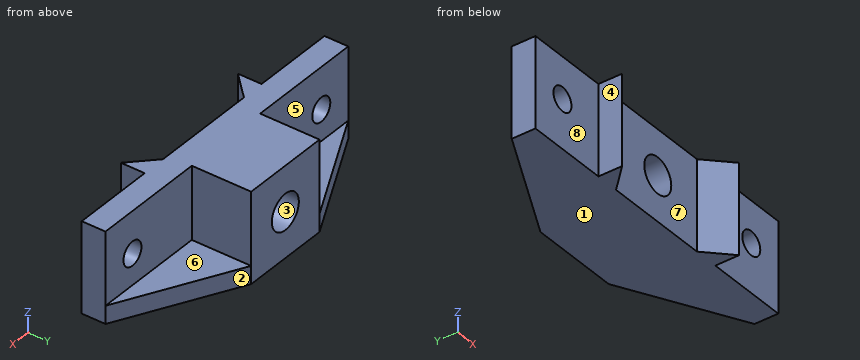
from build123d import *

# Parameters (mm, degrees)
BOSS_EXTRUDE1_DEPTH = 76
CUT_EXTRUDE1_DEPTH  = 61
SKETCH7_R           = 15
SKETCH7_R_2         = 10
CUT_EXTRUDE4_DEPTH  = 71


with BuildPart() as part:
    # Sketch2 → Boss-Extrude1 (new body)
    with BuildSketch(Plane.XY):
        Polygon((155.98455698, -34.815353078), (57.98455698, -84.815353078), (57.98455698, -104.815353078), (127.98455698, -104.815353078), (127.98455698, -124.815353078), (147.58455698, -104.815353078), (237.576393715, -104.815353078), (257.98455698, -124.815353078), (257.98455698, -104.815353078), (327.98455698, -104.815353078), (327.98455698, -84.815353078), (231.98455698, -34.815353078), align=None)
    extrude(amount=BOSS_EXTRUDE1_DEPTH)

    # Sketch5 → Cut-Extrude1 (cut)
    with BuildSketch(Plane.XY.offset(76)):
        Polygon((155.98455698, -34.815353078), (155.98455698, -84.815353078), (57.98455698, -84.815353078), align=None)
        Polygon((231.98455698, -34.815353078), (231.98455698, -84.815353078), (327.98455698, -84.815353078), align=None)
    extrude(amount=-CUT_EXTRUDE1_DEPTH, mode=Mode.SUBTRACT)

    # Sketch7 → Cut-Extrude4 (cut, through all)
    with BuildSketch(Plane(origin=(0, -104.815353078, 0), x_dir=(1, 0, 0), z_dir=(0, 1, 0))):
        with Locations((193.98455698, -38)):
            Circle(SKETCH7_R)
        with Locations((87.98455698, -41)):
            Circle(SKETCH7_R_2)
        with Locations((297.98455698, -41)):
            Circle(SKETCH7_R_2)
    extrude(amount=CUT_EXTRUDE4_DEPTH, mode=Mode.SUBTRACT)


solid = part.part
Model file for the job. Use its own axes, mm. Face numbers are marked on the shaded views. A direction names the side the tool comes from. Give positions to 0.01 mm unless a question says otherwise; leave off trailing zeros. Order: outer loops, then holes, each group sorted by start corner. A loop starts at its lowest first (then second) coordinate and runs counter-clockwise, first axis right, second up. Notation, with made-up numbers: M 20,24 L 25,24 A27 cw 25,54 Z; hole C 36,64 d9. An arc over 180 degrees is marked long. Put each result on its own line as item: value. Start each with the question number.
(1) Tool access for the marked faces 5, 6, 7 and 8: list every direction of +Z, -Z, +X, -X, +Y, -Y with a clear straight run to the whole face (end or side of a thin tool).
(2) Band-saw the part on A-A on z = 9. Give the cut face in (x, y), then the cut area to 3 significant figures.
(3) Band-saw the part on B-B on x = 190. Give the cut face in (y, z), then the cut area to 3 significant figures.
(4) Drill centre lines: L1, parallel to X at y = -90.75, z = 41; L2, parallel to X at y = -98, z = 49.5; L3, parallel to X at y = -115.5, z = 37. Where is each one in solid material? Low to high. Write a range as [from, to].
(5) Pin check, flat tips, straight feed: pin 1 Ø22 at (y, z) = (-119, 29) entering from -X; pin 2 Ø5 at (x, z) = (262, 12.5) entering from -Y; pin 3 Ø8 at (x, z) = (252.5, 53.5) entering from +Y. Stop position of each tip, or through.
(6) Band-saw the part on C-C on y = -58.5. Give the cut face in (x, z), then the cut area to 3 significant figures.
(7) Band-saw the part on D-D on z = 48.5. Give the cut face in (x, y), then the cut area to 3 significant figures.
(8) Pull direction X, two halves, no side cores. Call the marked faces 1, 2, 3 and 4: released by +X, released by -X, zero draft, split by the parting line, or undercut.
Results below:
1. face 5: +Z, -X, +Y
1. face 6: +Z, +X, +Y
1. face 7: +Z, -Z, -Y
1. face 8: +Z, -Z, -X, -Y
2. outline: M 57.98,-104.82 L 127.98,-104.82 L 127.98,-124.82 L 147.58,-104.82 L 237.58,-104.82 L 257.98,-124.82 L 257.98,-104.82 L 327.98,-104.82 L 327.98,-84.82 L 231.98,-34.82 L 155.98,-34.82 L 57.98,-84.82 Z
2. area: 14,500 mm2
3. outline: M -104.82,0 L -34.82,0 L -34.82,23.54 L -104.82,23.54 Z; M -104.82,52.46 L -34.82,52.46 L -34.82,76 L -104.82,76 Z
3. area: 3,300 mm2
4. L1: x = [57.98, 77.98], [97.98, 179.29], [208.68, 287.98], [307.98, 327.98]
4. L2: x = [57.98, 82.72], [93.25, 184.35], [203.62, 292.72], [303.25, 327.98]
4. L3: x = [127.98, 137.11], [248.48, 257.98]
5. pin 1: stops at x = 127.98
5. pin 2: stops at y = -104.82
5. pin 3: stops at y = -84.82
6. outline: M 109.56,0 L 277.46,0 L 277.46,15 L 231.98,15 L 231.98,76 L 155.98,76 L 155.98,15 L 109.56,15 Z; hole C 193.98,38 d30
6. area: 6,450 mm2
7. outline: M 57.98,-104.82 L 81.37,-104.82 L 81.37,-84.82 L 57.98,-84.82 Z; M 94.6,-104.82 L 127.98,-104.82 L 127.98,-124.82 L 147.58,-104.82 L 183.27,-104.82 L 183.27,-34.82 L 155.98,-34.82 L 155.98,-84.82 L 94.6,-84.82 Z; M 204.7,-104.82 L 237.58,-104.82 L 257.98,-124.82 L 257.98,-104.82 L 291.37,-104.82 L 291.37,-84.82 L 231.98,-84.82 L 231.98,-34.82 L 204.7,-34.82 Z; M 304.6,-104.82 L 327.98,-104.82 L 327.98,-84.82 L 304.6,-84.82 Z
7. area: 7,570 mm2
8. face 1: zero draft
8. face 2: released by +X
8. face 3: undercut
8. face 4: released by -X
